Study the drawing (mm; zero at the part's minimum x, y, z) and answer. A direction names the side the tool comes from. Coordinates: 2 decimals unless noted, no trailing zeros. Order: outer loops, then holes, each group sorted by start corner. A loop starts at its lowest first (then second) coordinate and runs counter-clockwise, first axis right, second up. Notation, with made-up numbers: M 58,1 L 84,1 A23 ccw 84,20 Z; hole C -39.5,63.25 d8. An arc over 180 degrees is marked long. Put each result on its own line as item: value.
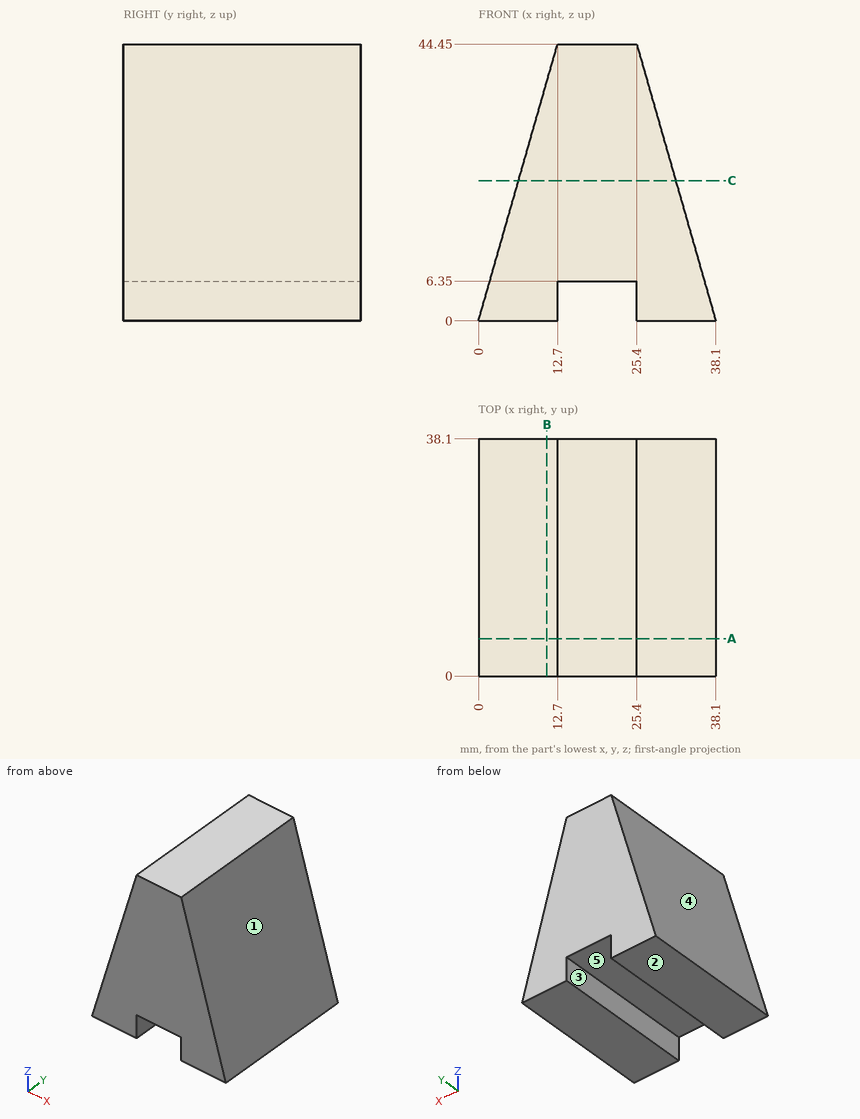
Q1. A tool of negligible diameter and unlimited length cuts with its end or side. For the marked faces 4 and 5, from which of +Z, -Z, +X, -X, +Y, -Y can it reach the whole face along a straight path? Write none if from no direction.
Answers below:
face 4: +Z, -X, +Y, -Y
face 5: -Z, +Y, -Y
Q2. Given pin 1 (4 mm diameter, centred on y = 19.5, z = 32, fed in from -X); pin 2 (1 mm diameter, centred on y = 21, z = 24, fed in from -X); pin 3 (1.9 mm diameter, centred on y = 14, z = 4.5, fed in from -X), each flat-ended and moving along its own axis, determine where each tip first touches the part or whether it passes through.
Answers below:
pin 1: stops at x = 8.57
pin 2: stops at x = 6.71
pin 3: stops at x = 1.01
Q3. Find section A-A on y = 6. Write down the section's boundary in (x, z).
Answers below:
outline: M 0,0 L 12.7,0 L 12.7,6.35 L 25.4,6.35 L 25.4,0 L 38.1,0 L 25.4,44.45 L 12.7,44.45 Z
Q4. Consider line 1 along Z through (x, y) = (15.5, 26.5); line 2 along X through (y, z) = (14, 24.5); line 3 along X through (y, z) = (2, 9.5). Determine where each line is inside the solid, lowest interval first.
Answers below:
line 1: z = 6.35 to 44.45
line 2: x = 7 to 31.1
line 3: x = 2.71 to 35.39
Q5. Find section C-C on z = 22.5. Write down the section's boundary in (x, y), plus the area to 3 significant figures.
Answers below:
outline: M 6.43,0 L 31.67,0 L 31.67,38.1 L 6.43,38.1 Z
area: 962 mm^2
Q6. Find section B-B on x = 11. Write down the section's boundary in (y, z), plus the area to 3 significant figures.
Answers below:
outline: M 0,0 L 38.1,0 L 38.1,38.5 L 0,38.5 Z
area: 1,470 mm^2
Q7. For a pull along X with two mould halves and no side action, classify the marked faces 1, 2 and 3 as +X half, -X half, draft (parallel to the pull), parting line (faces both ways), or undercut.
Answers below:
face 1: +X half
face 2: draft
face 3: undercut
